Read the model definition and answer for the solid it produces. Units are mm, in the model's axes. Coordinates: 2 decimals unless noted, no trailing zeros. Loops run counter-clockwise (first coordinate to the right, second up) from the corner with the lowest first, then second, coordinate; pieces in that order, holes last.
Autodesk Inventor part; units mm, degrees
ref_plane "YZ Plane" through (0, 0, 0) normal (1, 0, 0) x (0, 1, 0)
ref_plane "XZ Plane" through (0, 0, 0) normal (0, 1, 0) x (-1, 0, 0)
ref_plane "XY Plane" through (0, 0, 0) normal (0, 0, 1) x (1, 0, 0)
sketch "Sketch1" plane through (0, 0, 0) normal (0, 1, 0) x (-1, 0, 0)
  line L0 (-2.54, 0) -> (-27.94, 0)
  line L1 (-30.48, -16.51) -> (-30.48, -16.51)
  line L2 (-27.94, -19.05) -> (-2.54, -19.05)
  line L3 (0, -16.51) -> (0, -16.51)
  circle A0 centre (-2.54, -16.51) radius 1.016
  circle A1 centre (-27.94, -16.51) radius 1.016
  circle A2 centre (-2.54, -3.556) radius 1.016
  circle A3 centre (-27.94, -3.556) radius 1.016
  line L4 (-3.175, -19.05) -> (-27.305, -19.05)
  line L5 (-27.305, -19.05) -> (-27.305, 0)
  line L6 (-27.305, 0) -> (-3.175, 0)
  line L7 (-3.175, 0) -> (-3.175, -19.05)
  line L8 (-2.54, -13.97) -> (-27.94, -13.97)
  line L9 (-30.48, -13.97) -> (-30.48, -6.096)
  line L10 (-27.94, -6.096) -> (-2.54, -6.096)
  line L11 (0, -6.096) -> (0, -13.97)
  arc A4 (-2.54, -19.05) -> (0, -16.51) centre (-2.54, -16.51) ccw
  arc A5 (-30.48, -16.51) -> (-27.94, -19.05) centre (-27.94, -16.51) ccw
  arc A6 (0, -16.51) -> (-2.54, -13.97) centre (-2.54, -16.51) ccw
  arc A7 (-27.94, -13.97) -> (-30.48, -16.51) centre (-27.94, -16.51) ccw
  line L12 (0, -3.556) -> (0, -2.54)
  line L13 (-30.48, -3.556) -> (-30.48, -2.54)
  arc A8 (-30.48, -3.556) -> (-27.94, -6.096) centre (-27.94, -3.556) ccw
  arc A9 (-27.94, 0) -> (-30.48, -2.54) centre (-27.94, -2.54) ccw
  arc A10 (0, -2.54) -> (-2.54, 0) centre (-2.54, -2.54) ccw
  arc A11 (-2.54, -6.096) -> (0, -3.556) centre (-2.54, -3.556) ccw
  line L14 (-0.2121, -1.524) -> (-30.2679, -1.524) construction
  circle A12 centre (-5.08, -1.524) radius 0.508
  circle A13 centre (-7.62, -1.524) radius 0.508
  circle A14 centre (-10.16, -1.524) radius 0.508
  circle A15 centre (-12.7, -1.524) radius 0.508
  circle A16 centre (-15.24, -1.524) radius 0.508
  circle A17 centre (-17.78, -1.524) radius 0.508
  circle A18 centre (-20.32, -1.524) radius 0.508
  circle A19 centre (-22.86, -1.524) radius 0.508
  circle A20 centre (-25.4, -1.524) radius 0.508
  point P0 (0, 0)
  point P1 (-30.48, -19.05)
  point P2 (-30.48, 0)
  point P3 (0, -19.05)
  point P4 (-3.175, -13.97)
  point P5 (-3.175, -6.096)
  point P6 (-27.305, -6.096)
  point P7 (-27.305, -13.97)
  dimension "d0" = 30.48
  dimension "d1" = 19.05
  dimension "d2" = 3.556
  dimension "d3" = 3.556
  dimension "d4" = 2.54
  dimension "d5" = 2.54
  dimension "d6" = 2.54
  dimension "d7" = 2.54
  dimension "d8" = 12.954
  dimension "d9" = 12.954
  dimension "d10" = 2.032
  dimension "d11" = 24.13
  dimension "d12" = 3.175
  dimension "d13" = 3.175
  dimension "d14" = 2.54
  dimension "d15" = 2.54
  dimension "d16" = 2.54
  dimension "d17" = 2.54
  dimension "d18" = 1.524
  dimension "d19" = 5.08
  dimension "d22" = 2.54
  dimension "d27" = 5.08
  dimension "d28" = 1.016
  dimension "d31" = 2.54
extrude "Extrusion1" add sketch "Sketch1" along normal blind 1.6 contours A10 L12 A11 L10 L7 A2 L0 | L7 A2 L10 L5 A3 L0 | L5 A3 L10 A8 L13 A9 L0 | L7 L8 L5 L10 | L8 A6 A4 L2 L7 A0 | L7 A0 L2 L5 A1 L8 | L5 A1 L2 A5 A7 L8
equation "\"d12\" = d13"
properties part number "L3GD20H footprint"
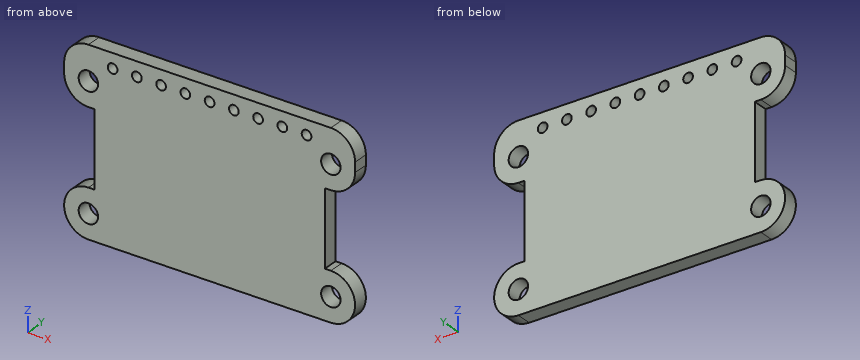
Item 1: Given pin 1 (3.5 mm diameter, centred on x = 27.94, z = -16.51, fed in from -Y); pin 2 (0.9 mm diameter, centred on x = 7.62, z = -1.524, fed in from -Y); pin 3 (0.5 mm diameter, centred on y = 1, z = -8, fed in from +X) (3 decimals), each flat-ended and moving along its own axis, determine where each tip first touches the part or whether it passes through.
Numbers:
pin 1: stops at y = 0
pin 2: passes through
pin 3: stops at x = 27.305
Item 2: Find the intervals of material crossed by line 1 along Z through (x, y) = (27.94, 0.55); line 2 along Z through (x, y) = (10.16, 0.9); line 3 along X through (y, z) = (1.1, -3.75), in increasing order.
Numbers:
line 1: z = -19.05 to -17.53, -15.49 to -13.97, -6.1 to -4.57, -2.54 to 0
line 2: z = -19.05 to -2.03, -1.02 to 0
line 3: x = 0.01 to 1.54, 3.54 to 26.94, 28.94 to 30.47
Item 3: A cutting plane is placed at B-B on z = -3. Determine the outline of the cut face in (x, y).
Numbers:
outline: (0, 0) - (1.69, 0) - (1.69, 1.6) - (0, 1.6) - close; (3.39, 0) - (27.09, 0) - (27.09, 1.6) - (3.39, 1.6) - close; (28.79, 0) - (30.48, 0) - (30.48, 1.6) - (28.79, 1.6) - close
Item 4: A cutting plane is placed at A-A on x = 17.78. Determine the outline of the cut face in (y, z), then the cut area to 3 significant figures.
Numbers:
outline: (0, -19.05) - (1.6, -19.05) - (1.6, -2.03) - (0, -2.03) - close; (0, -1.02) - (1.6, -1.02) - (1.6, 0) - (0, 0) - close
area: 28.9 mm2
Item 5: A cutting plane is placed at C-C on x = 7.5. Determine the outline of the cut face in (y, z).
Numbers:
outline: (0, -19.05) - (1.6, -19.05) - (1.6, -2.02) - (0, -2.02) - close; (0, -1.03) - (1.6, -1.03) - (1.6, 0) - (0, 0) - close
Item 6: A cutting plane is placed at D-D on y = 1.15. Give the number of separate pieces and of enclosed holes in the cut face, then the cut area to 3 significant figures.
Numbers:
separate pieces: 1
enclosed holes: 13
area: 499 mm2
